Here's how the part is built. I have some questions about the finished solid (model axes, mm). A direction names the side the tool comes from. Round coordinates to 2 decimals unless told otherwise and drop trailing zeros. Order: outer loops, then holes, each group sorted by start corner. A loop starts at its lowest first (then second) coordinate and runs counter-clockwise, first axis right, second up.
```python
from build123d import *

# Parameters (mm, degrees)
F1_DEPTH = 25.4
F2_DEPTH = 205.74
F3_R     = 5.08


with BuildPart() as f1:
    # F0 (on Front) → F1 (new body)
    with BuildSketch(Plane.XZ):
        with BuildLine():
            Line((-137.8654783239, -94.8646968782), (-137.8654783239, 77.1448463202))
            add(Edge.make_bspline(
                [(-137.8654783239, -94.8646968782), (-158.2706578332, -91.8585594164), (-166.981581766, -7.7451420633), (-156.4983493038, 60.4911413287), (-137.8654783239, 77.1448463202)],
                knots=[0.5687155023, 0.5687155023, 0.5687155023, 0.5687155023, 0.6668544702, 0.7702510453, 0.7702510453, 0.7702510453, 0.7702510453], degree=3))
        make_face()
        with BuildLine():
            add(Edge.make_bspline(
                [(-137.8654783239, 77.1448463202), (-118.4092236957, 94.5344759251), (-46.2534441965, 88.953036709), (88.0846333213, 108.6653008956), (92.4056395888, 77.1448463202)],
                knots=[0.7702510453, 0.7702510453, 0.7702510453, 0.7702510453, 0.8782166988, 1, 1, 1, 1], degree=3))
            Line((-137.8654783239, 77.1448463202), (92.4056395888, 77.1448463202))
        make_face()
        with BuildLine():
            Line((92.4056395888, 77.1448463202), (-137.8654783239, 77.1448463202))
            Line((-137.8654783239, 77.1448463202), (-137.8654783239, -94.8646968782))
            Line((-137.8654783239, -94.8646968782), (-132.5711192259, -94.8646968782))
            add(Edge.make_bspline(
                [(92.4056395888, 70.2900443589), (88.177524096, 33.099393391), (0.8242697931, -63.9641826889), (-13.3528421954, -30.7865615999), (4.0839060304, -11.2757699491), (44.4742754931, 31.0623950536), (-38.227277915, 53.3707628282), (-31.9830279818, -8.9984561018), (-106.4943951176, -91.5314031198), (-132.5711192259, -94.8646968782)],
                knots=[0.0081423274, 0.0081423274, 0.0081423274, 0.0081423274, 0.1316241862, 0.1715089751, 0.2275439291, 0.2959483496, 0.3705997718, 0.4486594468, 0.560717639, 0.560717639, 0.560717639, 0.560717639], degree=3))
            Line((92.4056395888, 70.2900443589), (92.4056395888, 77.1448463202))
        make_face()
        with BuildLine():
            Line((92.4056395888, -44.0646968782), (92.4056395888, 70.2900443589))
            add(Edge.make_bspline(
                [(92.4056395888, 70.2900443589), (88.177524096, 33.099393391), (0.8242697931, -63.9641826889), (-13.3528421954, -30.7865615999), (4.0839060304, -11.2757699491), (44.4742754931, 31.0623950536), (-38.227277915, 53.3707628282), (-31.9830279818, -8.9984561018), (-106.4943951176, -91.5314031198), (-132.5711192259, -94.8646968782)],
                knots=[0.0081423274, 0.0081423274, 0.0081423274, 0.0081423274, 0.1316241862, 0.1715089751, 0.2275439291, 0.2959483496, 0.3705997718, 0.4486594468, 0.560717639, 0.560717639, 0.560717639, 0.560717639], degree=3))
            Line((-132.5711192259, -94.8646968782), (41.6056395888, -94.8646968782))
            ThreePointArc((41.6056395888, -94.8646968782), (77.5266640731, -79.9857213625), (92.4056395888, -44.0646968782))
        make_face()
    extrude(amount=F1_DEPTH)

    # F2 (add): a face of the model
    f2_faces = [f1.faces().sort_by_distance(p)[0] for p in [
        (-48.1299193675, -12.7, -94.8646968782),
    ]]
    extrude(f2_faces, amount=F2_DEPTH)

    # F3
    f3_edges = [f1.edges().sort_by_distance(p)[0] for p in [
        (41.60564, -12.7, -300.604697),
        (-137.865478, -12.7, -300.604697),
    ]]
    fillet(f3_edges, radius=F3_R)


solid = f1.part
```
1) I need wall thicknesses on line 1 (X direction, y = -19.25, z = -139.5); line 2 (Z direction, x = 25, y = -4.25); line 3 (X direction, y = -1.5, z = 74.5). Which ranges of each line are inside material? Lowest first, please.
2) If we section it at A-A (z = -107): Write out the boundary of the cut face in (x, y), plus the area to 3 significant figures.
3) We'd pull the mould along Y, two halves only. Please class faces 1 (the flat face through (-39, -25.4, -93)), 2 (the flat face through (41.606, -13, -194)), 3 (the flat face through (-39, 0, -93)): +Y half, -Y half, draft (parallel to the pull), parting line (faces both ways), or undercut.
4) For faces 4 (the cylindrical face through (77.13, -12.52, -80.38)), 5 (the flat face through (-137.865, -13, -194)), which set-ups out of +Z, -Z, +X, -X, +Y, -Y let a thin tool reach every point of the face, with its end or its side?
5) I'm going to push flat-ended pins straight in: pin 1 (1 mm diameter, centred on y = -11.5, z = -105, fed in from -X); pin 2 (1.5 mm diameter, centred on x = -8, y = -4, fed in from +Z); pin 3 (12 mm diameter, centred on x = -9, y = -3, fed in from +Z). Where does each tip first touch, or does it pass through?
Solutions:
1. line 1: x = -137.87 to 41.61
1. line 2: z = -300.6 to 98.99
1. line 3: x = -140.57 to 92.41
2. outline: (-137.87, -25.4) - (41.61, -25.4) - (41.61, 0) - (-137.87, 0) - close
2. area: 4,560 mm2
3. face 1: -Y half
3. face 2: draft
3. face 3: +Y half
4. face 4: -Z, +X, +Y, -Y
4. face 5: -Z, -X, +Y, -Y
5. pin 1: stops at x = -137.87
5. pin 2: stops at z = 97.04
5. pin 3: stops at z = 97.35
